Can you work these out from the drawing? Everything is in mm from the part's minimum corner. Coordinates: 2 decimals unless noted, no trailing zeros. Loops run counter-clockwise (first coordinate to the right, second up) from the corner with the lowest first, then second, coordinate; pieces in that order, holes last. Notation, with made-up numbers: (-12.75, 57) - (43.25, 57) arc R22 ccw to (43.25, 78) - close; hole circle Ø3 at (-12.75, -29.5). An arc over 180 degrees is marked (long way). Use CSV: the item, a comma, the result in double quotes.
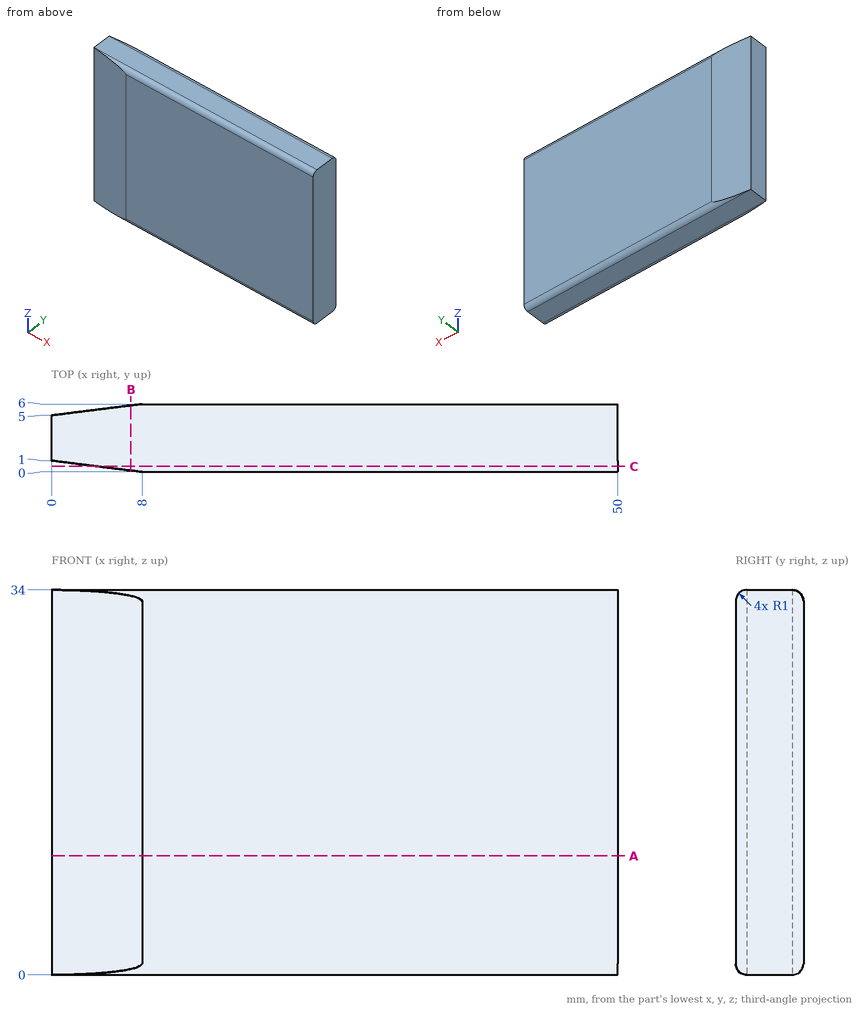
(1) Please list where these lines run through material, in increasing order: line 1 (Z direction, x = 36.5, y = 5.05); line 2 (Z direction, x = 33, y = 0.4).
Computed:
line 1,"z = 0 to 34"
line 2,"z = 0.2 to 33.8"
(2) Suppose I cut it at B-B (x = 7). Write out the boundary of the cut face in (y, z) (3 decimals).
Computed:
outline,"(0.125, 0.516) arc R1 ccw to (1, 0) - (5, 0) arc R1 ccw to (5.875, 0.516) - (5.875, 33.484) arc R1 ccw to (5, 34) - (1, 34) arc R1 ccw to (0.125, 33.484) - close"
(3) Suppose I cut it at A-A (z = 10.5). Write out the boundary of the cut face in (x, y).
Computed:
outline,"(0, 1) - (8, 0) - (50, 0) - (50, 6) - (8, 6) - (0, 5) - close"
(4) Suppose I cut it at C-C (y = 0.5). Write out the boundary of the cut face in (x, z), plus the area to 3 significant figures.
Computed:
outline,"(4, 0.13) - (50, 0.13) - (50, 33.87) - (4, 33.87) - close"
area,"1,550 mm²"
